```python
from build123d import *

# Parameters (mm, degrees)
F0_W           = 67
F0_H           = 5
F1_DEPTH       = 12
F2_DEPTH       = 43
F5_DEPTH       = 9
F6_W           = 5
F6_H           = 42
F7_DEPTH       = 100
F9_D           = 5
F9_CSINK_D     = 14
F9_CSINK_ANGLE = 45
F10_R          = 3


# Not quite as in the source:
# - a feature names something its author has since deleted; it is built from what else it names


with BuildPart() as f1:
    # F0 (on Top) → F1 (new body)
    with BuildSketch(Plane.XY):
        Polygon((57, -8), (0, -8), (57, -60), align=None)
        Polygon((67, 0), (0, 0), (0, -8), (57, -8), (57, -60), (67, -60), align=None)
        with Locations((33.5, 2.5)):
            Rectangle(F0_W, F0_H)
    extrude(amount=-F1_DEPTH)

    # F0 (on Top) → F2 (join)
    with BuildSketch(Plane.XY):
        Polygon((67, 0), (0, 0), (0, -8), (57, -8), (57, -60), (67, -60), align=None)
        with Locations((33.5, 2.5)):
            Rectangle(F0_W, F0_H)
    extrude(amount=F2_DEPTH)

    # F4 (on mid) → F5 (join, symmetric)
    with BuildSketch(Plane(origin=(62, 0, 0), x_dir=(0, -1, 0), z_dir=(-1, 0, 0))):
        with BuildLine():
            Line((42, 33), (29, 33))
            ThreePointArc((29, 33), (21, 25), (29, 17))
            Line((29, 17), (42, 17))
            ThreePointArc((42, 17), (50, 25), (42, 33))
        make_face()
        with BuildLine():
            ThreePointArc((42, 30), (47, 25), (42, 20))
            Line((42, 20), (29, 20))
            ThreePointArc((29, 20), (24, 25), (29, 30))
            Line((29, 30), (42, 30))
        make_face(mode=Mode.SUBTRACT)
    extrude(amount=F5_DEPTH, both=True)

    # F6 (on mid) → F7 (cut, symmetric)
    with BuildSketch(Plane(origin=(62, 0, 0), x_dir=(0, -1, 0), z_dir=(-1, 0, 0))):
        with BuildLine():
            ThreePointArc((43, 43), (55.0208152802, 38.0208152802), (60, 26))
            Line((60, 26), (60, 43))
            Line((60, 43), (43, 43))
        make_face()
        with BuildLine():
            Line((42, 30), (29, 30))
            ThreePointArc((29, 30), (24, 25), (29, 20))
            Line((29, 20), (42, 20))
            ThreePointArc((42, 20), (47, 25), (42, 30))
        make_face()
        with Locations((-2.5, 9)):
            Rectangle(F6_W, F6_H)
    extrude(amount=F7_DEPTH, both=True, mode=Mode.SUBTRACT)

    # F9 (through all)
    with Locations(Plane.XZ.offset(8)):
        with Locations((13, 18), (44, 18)):
            CounterSinkHole(F9_D / 2, F9_CSINK_D / 2, counter_sink_angle=F9_CSINK_ANGLE)

    # F10
    f10_edges = [f1.edges().sort_by_distance(p)[0] for p in [
        (57, -21, 25),
        (57, -35.5, 33),
        (57, -34, 0),
        (28.5, -8, 0),
        (57, -8, 21.5),
        (0, -1.5, 43),
    ]]
    fillet(f10_edges, radius=F10_R)


solid = f1.part
```
Geometry: final body of the model. Coordinates: model frame, mm. A direction names the side the tool comes from. Round coordinates to 2 decimals unless told otherwise and drop trailing zeros. Order: outer loops, then holes, each group sorted by start corner. A loop starts at its lowest first (then second) coordinate and runs counter-clockwise, first axis right, second up. Notation, with made-up numbers: (54, 56) -> (88, 56) arc R21 ccw to (88, 62) -> close; hole circle Ø4 at (37.5, 89). An arc over 180 degrees is marked (long way). Use one line per item in the form item = value. Start each with the question number.
1. Cut plane A-A (y = -5). Return the cut outline in (x, z).
2. Cut plane D-D (x = 52). Return the cut outline in (y, z), then the cut area to 3 significant figures.
3. Cut plane B-B (x = 44). Return the cut outline in (y, z), then the cut area to 3 significant figures.
4. Cut plane C-C (y = -30). Return the cut outline in (x, z).
5. Reachability of faces 4 (the face through (27.38, -8.86, 0.9)), 5 (the face through (62, -47, 25)), 6 (the face through (53.493, -21.002, 25.176)), 7 (the face through (56.14, -35.59, 16.1)) from +Z, -Z, +X, -X, +Y, -Y: full face, straight path, thin tool, end or side. Return the list, or none.
6. Line query: probe 1 along Z at (x, y) = (50, -27); probe 2 along Z at (x, y) = (56.5, 1); probe 3 along X at (y, z) = (-41.5, 3.5). Output: solid intervals per line, ascending.
7. Pin query (flat end, axial travel): pin 1 Ø4.5 at (x, y) = (70, -34.5) entering from -Z; pin 2 Ø1.1 at (x, y) = (53.5, -36) entering from +Z; pin 3 Ø16.5 at (y, z) = (-17, 11.5) entering from +X. Return the tip coordinate at first contact, or that it passes through.
8. Draft query along Z for faces 1 (the face through (69, -36, 33)), 2 (the face through (62, -24, 25)), 3 (the face through (71, -35.3, 30.4)). Return one class per face: pulls with the +Z half, pulls with the -Z half, needs draft (parallel to the pull), parting line crosses it, or undercut.
Solution:
q1.outline = (0, -12) -> (67, -12) -> (67, 43) -> (3, 43) arc R3 ccw to (0, 40) -> close; hole circle Ø11.51 at (13, 18); hole circle Ø11.51 at (44, 18)
q2.outline = (-55.44, -12) -> (0, -12) -> (0, 30) -> (5, 30) -> (5, 43) -> (-8, 43) -> (-8, 3) arc R3 cw to (-11, 0) -> (-55.44, 0) -> close
q2.area = 1,080 mm^2
q3.outline = (-48.14, -12) -> (0, -12) -> (0, 14.31) -> (-8, 11) -> (-8, 3) arc R3 cw to (-11, 0) -> (-48.14, 0) -> close; (-8, 25) -> (0, 21.69) -> (0, 30) -> (5, 30) -> (5, 43) -> (-8, 43) -> close
q3.area = 903 mm^2
q4.outline = (24.12, -12) -> (67, -12) -> (67, 17) -> (71, 17) -> (71, 20) -> (53, 20) -> (53, 17) -> (54, 17) arc R3 cw to (57, 14) -> (57, 3) arc R3 cw to (54, 0) -> (24.12, 0) -> close; (53, 30) -> (71, 30) -> (71, 33) -> (67, 33) -> (67, 43) -> (57, 43) -> (57, 36) arc R3 cw to (54, 33) -> (53, 33) -> close
q5.face_4 = +Z, -X, -Y
q5.face_5 = +X, -X
q5.face_6 = -X
q5.face_7 = -X, -Y
q6.probe_1 = -12 to 0
q6.probe_2 = 30 to 43
q6.probe_3 = 57 to 67
q7.pin_1 = 17
q7.pin_2 = 33
q7.pin_3 = 67
q8.face_1 = pulls with the +Z half
q8.face_2 = undercut
q8.face_3 = needs draft
